Source: three-view drawing plus pictorial views. Frame: mm from the lowest corner of the part. A direction names the side the tool comes from. Coordinates: 2 decimals unless noted, no trailing zeros. Write each loop counter-clockwise with the first axis right and the second up, starting at its lowest first coordinate (ties: lowest second). Pieces come first, ordered by that corner, then holes. Notation, with made-up numbers: (-19, 45) -> (32, 45) arc R6 cw to (32, 51) -> close; hole circle Ø10 at (27.5, 73.25). An arc over 180 degrees is marked (long way). Write item = value, one per line.
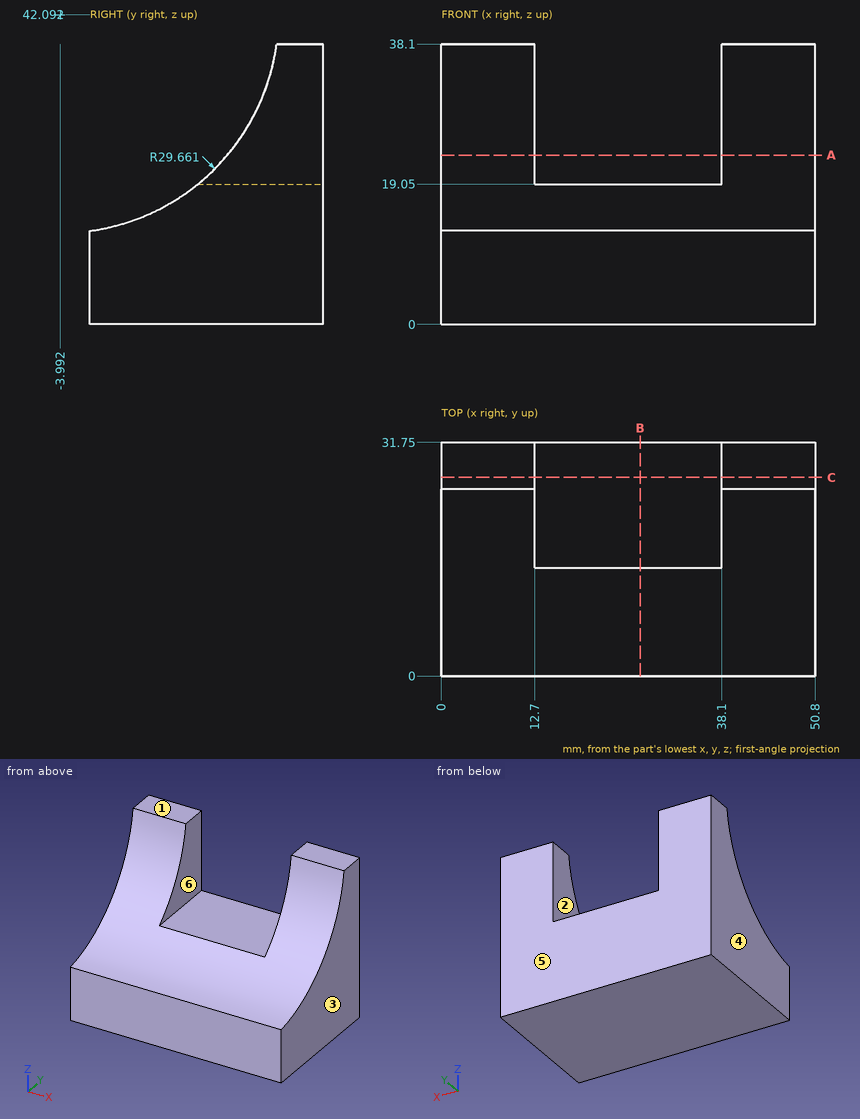
1) Cut plane C-C, the plane y = 27. Output: boundary loops of the cut face in (x, z), and give its area (3 significant figures).
Answer block:
outline = (0, 0) -> (50.8, 0) -> (50.8, 38.1) -> (38.1, 38.1) -> (38.1, 19.05) -> (12.7, 19.05) -> (12.7, 38.1) -> (0, 38.1) -> close
area = 1,450 mm2
2) First-contact query: pin 1 Ø13.5 at (x, y) = (27.5, 21.5) entering from +Z. Flat tip, straight axial feed; report the tip coordinate or a pass-through.
Answer block:
pin_1 = 19.05
3) Reachability of the marked faces 1 and 2 from +Z, -Z, +X, -X, +Y, -Y: full face, straight path, thin tool, end or side. Return the list, or none.
Answer block:
face_1 = +Z, +X, -X, +Y, -Y
face_2 = +Z, +Y, -Y
4) Pull-direction query (X, two-part tool) for the marked faces 3, 4, 5 and 6; classes: +X half, -X half, draft (parallel to the pull), parting line (faces both ways), or undercut.
Answer block:
face_3 = +X half
face_4 = -X half
face_5 = draft
face_6 = undercut
5) Cut plane A-A, the plane z = 23. Output: boundary loops of the cut face in (x, y).
Answer block:
outline = (0, 18.71) -> (12.7, 18.71) -> (12.7, 31.75) -> (0, 31.75) -> close; (38.1, 18.71) -> (50.8, 18.71) -> (50.8, 31.75) -> (38.1, 31.75) -> close
6) Cut plane B-B, the plane x = 27. Output: boundary loops of the cut face in (y, z).
Answer block:
outline = (0, 0) -> (31.75, 0) -> (31.75, 19.05) -> (14.69, 19.05) arc R29.66 cw to (0, 12.7) -> close
7) Material intervals for probe 1 along X at (y, z) = (29, 34); probe 2 along Z at (x, y) = (19, 24); probe 3 along Z at (x, y) = (22, 4), sorted ascending. Write a range as [from, to].
Answer block:
probe_1 = [0, 12.7], [38.1, 50.8]
probe_2 = [0, 19.05]
probe_3 = [0, 13.53]
